```python
from build123d import *

# Parameters (mm, degrees)
BOSS_EXTRUDE2_DEPTH = 5
SKETCH2_R           = 2.875
BOSS_EXTRUDE3_DEPTH = 5


with BuildPart() as part:
    # Sketch1 → Boss-Extrude2 (new body)
    with BuildSketch(Plane.XY):
        Polygon((0, 5), (45, 5), (45, -5), (-45, -5), (-45, 5), align=None)
    extrude(amount=-BOSS_EXTRUDE2_DEPTH)

    # Sketch2 → Boss-Extrude3 (add)
    with BuildSketch(Plane.XY):
        with Locations(Location((0, 0, 0), (0, 0, 180))):
            Circle(SKETCH2_R)
    extrude(amount=BOSS_EXTRUDE3_DEPTH)


solid = part.part
```
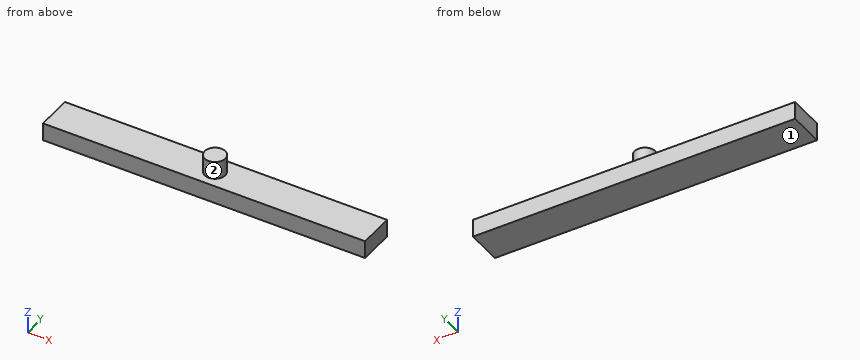
Part model, mm, in its own coordinate system. Face numbers are marked on the shaded views. A direction names the side the tool comes from. Round coordinates to 2 decimals unless told otherwise and drop trailing zeros. Write each loop counter-clockwise with the first axis right and the second up, starting at its lowest first coordinate (ties: lowest second). Pieces come first, ordered by that corner, then holes. Notation, with made-up numbers: M 10,33.5 L 60,33.5 A16 ccw 60,42.5 Z; hole C -7,-33.5 d7. An arc over 180 degrees is marked long. Answer as CSV lines item,"result". Start each with the question number.
1) Which spindle directions (+Z, -Z, +X, -X, +Y, -Y) get a long thin tool onto all of the face, cutting with end or side? Do the marked faces 1 and 2. Say none if no direction does.
2) Band-saw the part on A-A (x = 0). List the corners of the cut face in (y, z) (3 decimals), then the cut area to 4 significant figures.
3) Band-saw the part on D-D (x = 20). List the corners of the cut face in (y, z).
4) Drop a flat-ended pin along its axis: pin 1 (3 mm diameter, centred on x = 30, z = 2.5, fed in from -Y). Give the stop position or say it passes through.
5) Band-saw the part on C-C (z = 1.25). List the corners of the cut face in (x, y) (3 decimals), then the cut area to 3 significant figures.
6) Drill centre lines: L1, parallel to Z at x = 18, y = -0.75; L2, parallel to X at y = 1.25, z = 4. Where is each one in solid material? Low to high.
7) Band-saw the part on B-B (y = 0). List the corners of the cut face in (x, z) (3 decimals).
Worked out:
1,face 1,"-Z, +X, -X, +Y, -Y"
1,face 2,"+Z"
2,outline,"M -5,-5 L 5,-5 L 5,0 L 2.875,0 L 2.875,5 L -2.875,5 L -2.875,0 L -5,0 Z"
2,area,"78.75 mm²"
3,outline,"M -5,-5 L 5,-5 L 5,0 L -5,0 Z"
4,pin 1,"through"
5,outline,"C 0,0 d5.75"
5,area,"26.0 mm²"
6,L1,"-5 to 0"
6,L2,"-2.59 to 2.59"
7,outline,"M -45,-5 L 45,-5 L 45,0 L 2.875,0 L 2.875,5 L -2.875,5 L -2.875,0 L -45,0 Z"
